Design review of the part built by this model. Coordinates are the model's own, in mm. A direction names the side the tool comes from. Round coordinates to 2 decimals unless told otherwise and drop trailing zeros. Write each loop counter-clockwise with the first axis right and the second up, starting at its lowest first coordinate (ties: lowest second). Pieces come first, ordered by that corner, then holes. Notation, with made-up numbers: M -39,-37 L 12,-37 A20 cw 12,-30 Z; hole C 26.25,64 d9. An arc over 180 degrees is marked long. Use CSV: the item, a comma, the result in double quotes.
from build123d import *

# Parameters (mm, degrees)
F0_W     = 26
F0_H     = 50
F1_DEPTH = 25
F3_W     = 5
F3_H     = 50
F4_DEPTH = 5
F5_R     = 1.5
F6_DEPTH = 25
F2_W     = 1
F2_H     = 8.4868058562
F7_DEPTH = 77.6
F8_W     = 40
F8_H     = 5
F9_DEPTH = 25


with BuildPart() as f1:
    # F0 (on Top) → F1 (new body)
    with BuildSketch(Plane.XY):
        Rectangle(F0_W, F0_H)
    extrude(amount=F1_DEPTH)

    # F3 (on face) → F4 (join)
    with BuildSketch(Plane.XY.offset(25)):
        Rectangle(F3_W, F3_H)
    extrude(amount=F4_DEPTH)

    # F5 (on face) → F6 (cut)
    with BuildSketch(Plane.YZ.offset(2.5)):
        with Locations((-22.5, 27.5)):
            Circle(F5_R)
        with Locations((22.5, 27.5)):
            Circle(F5_R)
    extrude(amount=-F6_DEPTH, mode=Mode.SUBTRACT)

    # F2 (on face) → F7 (cut)
    with BuildSketch(Plane.XZ.offset(25)):
        Polygon((-5, 7.5), (5, 7.5), (5, 17.5), (0.5, 17.5), (-0.5, 17.5), (-5, 17.5), align=None)
        Polygon((0.5, 17.5), (5, 17.5), (0.5, 22), align=None)
        Polygon((-0.5, 22), (-5, 17.5), (-0.5, 17.5), align=None)
        with Locations((0, 29.2434029281)):
            Rectangle(F2_W, F2_H)
        Polygon((-0.5, 17.5), (0.5, 17.5), (0.5, 22), (0.5, 25), (-0.5, 25), (-0.5, 22), align=None)
        Polygon((13, 25), (9.4331367873, 25), (9.4331367873, 2.3707551882), (9.4331367873, 0), (13, 0), align=None)
        Polygon((-9.4218887389, 2.3707551882), (-9.4218887389, 25), (-13, 25), (-13, 0), (9.4331367873, 0), (9.4331367873, 2.3707551882), align=None)
    extrude(amount=-F7_DEPTH, mode=Mode.SUBTRACT)

    # F8 (on face) → F9 (cut)
    with BuildSketch(Plane.YZ.offset(2.5)):
        with Locations((0, 27.5)):
            Rectangle(F8_W, F8_H)
    extrude(amount=-F9_DEPTH, mode=Mode.SUBTRACT)


solid = f1.part
1) Add section A-A on y = -22.5. Write out the cut boundary in (x, z).
Answers:
outline,"M -9.42,2.37 L 9.43,2.37 L 9.43,25 L 2.5,25 L 2.5,26 L 0.5,26 L 0.5,22 L 5,17.5 L 5,7.5 L -5,7.5 L -5,17.5 L -0.5,22 L -0.5,26 L -2.5,26 L -2.5,25 L -9.42,25 Z; M -2.5,29 L -0.5,29 L -0.5,30 L -2.5,30 Z; M 0.5,29 L 2.5,29 L 2.5,30 L 0.5,30 Z"
2) Machinability: for faces 1 (the face through (-5, 0, 13)), 2 (the face through (2, -20, 27)), 3 (the face through (2.5, -21, 26)), 4 (the face through (0.5, 0, 24)), 5 (the face through (-2.5, 24, 26)), which of the approach directions +Z, -Z, +X, -X, +Y, -Y give a long, thin tool a straight path to every point of the face, cutting with its end or side? Answer none if there is none.
Answers:
face 1,"+Y, -Y"
face 2,"+Z, +X, -X"
face 3,"+Z, +X, +Y, -Y"
face 4,"+Z, +Y, -Y"
face 5,"+Z, -X, +Y, -Y"
3) The part is to be moulded in two halves that separate along Y. For faces 6 (the face through (6, -25, 13)), 7 (the face through (-2, -22, 30)), 8 (the face through (-1, -20, 27)), say which applies: released by +Y, released by -Y, zero draft, split by the parting line, or undercut.
Answers:
face 6,"released by -Y"
face 7,"zero draft"
face 8,"undercut"
4) Add section D-D on x = -3. Write out the cut boundary in (y, z).
Answers:
outline,"M -25,2.37 L 25,2.37 L 25,7.5 L -25,7.5 Z; M -25,19.5 L 25,19.5 L 25,25 L -25,25 Z"
5) For pin 1 Ø10 at (x, y) = (-3.5, -2) entering from +Z; pin 2 Ø9 at (y, z) = (4, 26.5) entering from +X; pin 3 Ø3.5 at (y, z) = (22.5, 27.5) entering from +X; pin 4 Ø2.5 at (y, z) = (23, 28.5) entering from -X, all flat-tipped, find the tip position at first contact; note any pin that passes through.
Answers:
pin 1,"z = 25"
pin 2,"x = 9.43"
pin 3,"x = 2.5"
pin 4,"x = -2.5"
6) Add section B-B on x = 1. Write out the cut boundary in (y, z).
Answers:
outline,"M -25,2.37 L 25,2.37 L 25,7.5 L -25,7.5 Z; M -25,21.5 L 25,21.5 L 25,30 L 20,30 L 20,25 L -20,25 L -20,30 L -25,30 Z; hole C -22.5,27.5 d3; hole C 22.5,27.5 d3"
7) Add section C-C on z = 25.5. Write out the cut boundary in (x, y).
Answers:
outline,"M -2.5,-25 L -0.5,-25 L -0.5,-20 L -2.5,-20 Z; M -2.5,20 L -0.5,20 L -0.5,25 L -2.5,25 Z; M 0.5,-25 L 2.5,-25 L 2.5,-20 L 0.5,-20 Z; M 0.5,20 L 2.5,20 L 2.5,25 L 0.5,25 Z"
8) Wall thickness on line 1 along X through (y, z) = (-21.5, 8.75); line 2 along Z through (x, y) = (1.5, 17); line 3 along Z through (x, y) = (-1.4, 22.5): over which ranges is each line inside the solid? List them lowest first. Write a range as [from, to].
Answers:
line 1,"[-9.42, -5], [5, 9.43]"
line 2,"[2.37, 7.5], [21, 25]"
line 3,"[2.37, 7.5], [21.1, 26], [29, 30]"
